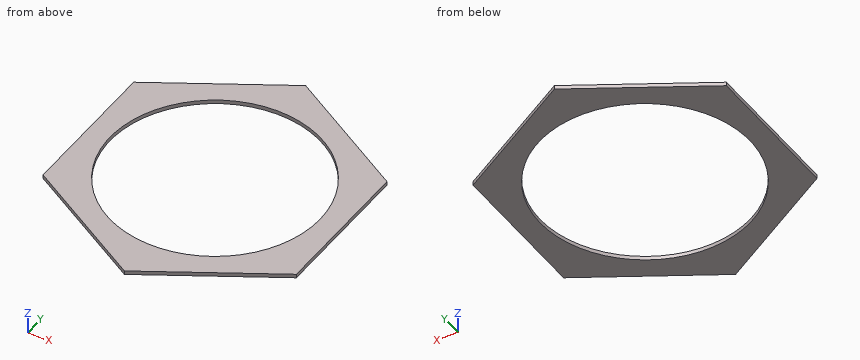
Autodesk Inventor part; units mm, degrees
ref_plane "YZ Plane" through (0, 0, 0) normal (1, 0, 0) x (0, 1, 0)
ref_plane "XZ Plane" through (0, 0, 0) normal (0, 1, 0) x (-1, 0, 0)
ref_plane "XY Plane" through (0, 0, 0) normal (0, 0, 1) x (1, 0, 0)
sketch "Sketch8" plane through (0, 0, 0) normal (0, 0, 1) x (1, 0, 0)
  circle A0 centre (0, 0) radius 82
  line L0 (99, -57.1577) -> (0, -114.3154)
  line L1 (0, -114.3154) -> (-99, -57.1577)
  line L2 (-99, -57.1577) -> (-99, 57.1577)
  line L3 (-99, 57.1577) -> (0, 114.3154)
  line L4 (0, 114.3154) -> (99, 57.1577)
  line L5 (99, 57.1577) -> (99, -57.1577)
  dimension "d44" = 164
  dimension "d47" = 198
extrude "Plate3" add sketch "Sketch8" along normal blind 3
equation "\"d48\" = Thickness"
equation "\"BendRadius\" = Thickness"
equation "\"BendReliefWidth\" = Thickness"
equation "\"BendReliefDepth\" = 0.5 * Thickness"
equation "\"CornerReliefSize\" = 4 * Thickness"
equation "\"MinimumRemnant\" = 2 * Thickness"
equation "\"TransitionRadius\" = BendRadius"
equation "\"JacobiRadiusSize\" = BendRadius"
equation "\"GapSize\" = Thickness"
equation "\"Octaeder_side\" = d41"
equation "\"Octaeder_flange_lenth\" = d42"
properties part number "DSB 121 drain system reduce flange"
CAD build for the part. Positions are in the model's coordinates, mm. Round coordinates to 2 decimals unless told otherwise and drop trailing zeros. Order: outer loops, then holes, each group sorted by start corner. A loop starts at its lowest first (then second) coordinate and runs counter-clockwise, first axis right, second up. Notation, with made-up numbers: (56.5, -28.75) - (83.5, -28.75) arc R9 ccw to (83.5, -16.75) - close; hole circle Ø4 at (72.25, -13). An arc over 180 degrees is marked (long way). Use CSV: the item, a comma, the result in double quotes. Start each with the question number.
1) Saw through at C-C (z = 0.8). List the corners of the cut face in (x, y), and give its area (3 significant figures).
2) Saw through at D-D (y = -85.5). List the corners of the cut face in (x, z).
3) Saw through at B-B (y = 0). List the corners of the cut face in (x, z), and give its area (3 significant figures).
4) Saw through at A-A (x = -4). List the corners of the cut face in (y, z).
5) Wall check: L1, parallel to Y at x = 0, z = 1.5; L2, parallel to X at y = 55, z = 2.5; L3, parallel to Y at x = 30.5, z = 1.45. Give the ranges that are in metal, low to high. Write a range as [from, to].
Values follow:
1,outline,"(-99, -57.16) - (0, -114.32) - (99, -57.16) - (99, 57.16) - (0, 114.32) - (-99, 57.16) - close; hole circle Ø164 at (0, 0)"
1,area,"12,800 mm2"
2,outline,"(-49.91, 0) - (49.91, 0) - (49.91, 3) - (-49.91, 3) - close"
3,outline,"(-99, 0) - (-82, 0) - (-82, 3) - (-99, 3) - close; (82, 0) - (99, 0) - (99, 3) - (82, 3) - close"
3,area,"102 mm2"
4,outline,"(-112.01, 0) - (-81.9, 0) - (-81.9, 3) - (-112.01, 3) - close; (81.9, 0) - (112.01, 0) - (112.01, 3) - (81.9, 3) - close"
5,L1,"y = [-114.32, -82], [82, 114.32]"
5,L2,"x = [-99, -60.82], [60.82, 99]"
5,L3,"y = [-96.71, -76.12], [76.12, 96.71]"
